```python
from build123d import *

# Parameters (mm, degrees)
SKETCH1_R           = 1
SKETCH1_R_2         = 8.5
SKETCH1_W           = 10
SKETCH1_H           = 3
SKETCH1_W_2         = 2.7
SKETCH1_H_2         = 10
BOSS_EXTRUDE1_DEPTH = 3
FILLET1_R           = 5


with BuildPart() as part:
    # Sketch1 → Boss-Extrude1 (new body)
    with BuildSketch(Plane.XY):
        Polygon((-18.34, -7), (-26.67, -7), (-26.67, -10), (-36.67, -10), (-36.67, -7), (-45, -7), (-45, -10), (-55, -10), (-55, -7), (-55, 27), (10, 27), (10, -7), (9.99, -7), (9.99, -10), (-0.01, -10), (-0.01, -7), (-8.34, -7), (-8.34, -10), (-18.34, -10), align=None)
        with Locations((-42.5, 17.5)):
            Circle(SKETCH1_R, mode=Mode.SUBTRACT)
        with Locations((-9, 10)):
            Circle(SKETCH1_R_2, mode=Mode.SUBTRACT)
        with Locations(Location((-36, 10, 0), (0, 0, 180))):
            Circle(SKETCH1_R_2, mode=Mode.SUBTRACT)
        with Locations(Location((-2.5, 17.5, 0), (0, 0, 180))):
            Circle(SKETCH1_R, mode=Mode.SUBTRACT)
        with Locations((-2.5, 2.5)):
            Circle(SKETCH1_R, mode=Mode.SUBTRACT)
        with Locations(Location((-42.5, 2.5, 0), (0, 0, 180))):
            Circle(SKETCH1_R, mode=Mode.SUBTRACT)
        with BuildLine():
            Line((-27.5, 19.5), (-17.5, 19.5))
            ThreePointArc((-17.5, 19.5), (-15.5, 17.5), (-17.5, 15.5))
            Line((-17.5, 15.5), (-27.5, 15.5))
            ThreePointArc((-27.5, 15.5), (-29.5, 17.5), (-27.5, 19.5))
        make_face(mode=Mode.SUBTRACT)
        with Locations((-22.5, 1.5)):
            Rectangle(SKETCH1_W, SKETCH1_H, mode=Mode.SUBTRACT)
        with Locations((-50, 10)):
            Rectangle(SKETCH1_W_2, SKETCH1_H_2, mode=Mode.SUBTRACT)
        with Locations((5, 10)):
            Rectangle(SKETCH1_W_2, SKETCH1_H_2, mode=Mode.SUBTRACT)
    extrude(amount=BOSS_EXTRUDE1_DEPTH)

    # Fillet1
    fillet1_edges = [part.edges().sort_by_distance(p)[0] for p in [
        (-55, 27, 1.5),
        (10, 27, 1.5),
    ]]
    fillet(fillet1_edges, radius=FILLET1_R)


solid = part.part
```
Check sheet for the modelled part. Datum: model origin and axes. Units: mm. A direction names the side the tool comes from. Coordinates: 2 decimals unless noted, no trailing zeros. Loops run counter-clockwise (first coordinate to the right, second up) from the corner with the lowest first, then second, coordinate; pieces in that order, holes last.
1) Sectioned sample at D-D (x = -2.5). Record the boundary of the cut face in (y, z), and give its area (3 significant figures).
2) Sectioned sample at B-B (x = -9). Record the boundary of the cut face in (y, z), and give its area (3 significant figures).
3) Sectioned sample at C-C (x = -23). Record the boundary of the cut face in (y, z), and give its area (3 significant figures).
4) Access from +Z, -Z, +X, -X, +Y, -Y to the whole of each face (thin tool, end or side, straight path). Record for faces 1 (the face through (-55, 6, 1)), 2 (the face through (-48.65, 10, 1)), 3 (the face through (-26.67, -8, 1)).
5) Gauge pin test, flat ends, axial feed: pin 1 (10 mm diameter, centred on x = -9, y = 10, fed in from +Z); pin 2 (0.9 mm diameter, centred on x = -39, z = 1.5, fed in from -Y). Record the tip position at first contact, or that the pin passes through.
6) Material ranges on probe 1 along X at (y, z) = (1, 1.1); probe 2 along Y at (x, z) = (-42.5, 2.35); probe 3 along Y at (x, z) = (-3, 2.6), recorded low to high.
7) Sectioned sample at A-A (y = -8). Record the boundary of the cut face in (x, z), and give its area (3 significant figures).
Check sheet entries:
1. outline: (-7, 0) - (1.5, 0) - (1.5, 3) - (-7, 3) - close; (3.5, 0) - (4.52, 0) - (4.52, 3) - (3.5, 3) - close; (15.48, 0) - (16.5, 0) - (16.5, 3) - (15.48, 3) - close; (18.5, 0) - (27, 0) - (27, 3) - (18.5, 3) - close
1. area: 57.1 mm2
2. outline: (-10, 0) - (1.5, 0) - (1.5, 3) - (-10, 3) - close; (18.5, 0) - (27, 0) - (27, 3) - (18.5, 3) - close
2. area: 60.0 mm2
3. outline: (-7, 0) - (0, 0) - (0, 3) - (-7, 3) - close; (3, 0) - (15.5, 0) - (15.5, 3) - (3, 3) - close; (19.5, 0) - (27, 0) - (27, 3) - (19.5, 3) - close
3. area: 81.0 mm2
4. face 1: +Z, -Z, -X, +Y, -Y
4. face 2: +Z, -Z
4. face 3: +Z, -Z, -Y
5. pin 1: passes through
5. pin 2: stops at y = -7
6. probe 1: x = -55 to -27.5, -17.5 to 10
6. probe 2: y = -7 to 1.5, 3.5 to 4.52, 15.48 to 16.5, 18.5 to 27
6. probe 3: y = -7 to 1.63, 3.37 to 3.98, 16.02 to 16.63, 18.37 to 27
7. outline: (-55, 0) - (-45, 0) - (-45, 3) - (-55, 3) - close; (-36.67, 0) - (-26.67, 0) - (-26.67, 3) - (-36.67, 3) - close; (-18.34, 0) - (-8.34, 0) - (-8.34, 3) - (-18.34, 3) - close; (-0.01, 0) - (9.99, 0) - (9.99, 3) - (-0.01, 3) - close
7. area: 120 mm2
